Read the model definition and answer for the solid it produces. Units are mm, in the model's axes. Face numbers are marked on the shaded views. Coordinates: 2 decimals unless noted, no trailing zeros. Write each loop counter-clockwise with the first axis right and the second up, starting at its lowest first coordinate (ties: lowest second). Pieces come first, ordered by that corner, then holes.
1) The part is cut by section C-C (y = 56). Determine the outline of the cut face in (x, z).
2) Find the intervals of material crossed by line 1 (Y direction, x = 1.4, z = 8.2); line 2 (X direction, y = 48, z = 8.25); line 3 (Z direction, x = 15.25, y = 73), in increasing order.
3) Determine the mould class of the marked faces 1, 2, 3 and 4 for opening direction X: +X half, -X half, draft (parallel to the pull), parting line (faces both ways), or undercut.
4) Each of these flat-tipped pins is pushed along its axis until it touches: pin 1 Ø3.5 at (y, z) = (80, 8.2) entering from +X; pin 2 Ø1 at (x, z) = (26, 5.5) entering from +Y; pin 3 Ø1 at (x, y) = (22.5, 53) entering from +Z; pin 4 Ø1.6 at (x, z) = (25.5, 9.5) entering from -Y. Where does it stop, or does it pass through?
5) The part is cut by section A-A (z = 8.2). Determine the outline of the cut face in (x, y).
6) The part is cut by section D-D (x = 19). Determine the outline of the cut face in (y, z), then the cut area to 3 significant figures.
7) The part is cut by section B-B (y = 80). Determine the outline of the cut face in (x, z).
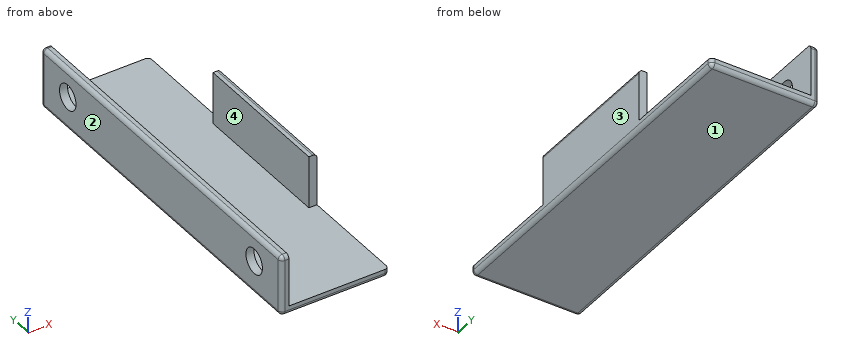
from build123d import *

# Parameters (mm, degrees)
SKETCH1_W           = 26.7
SKETCH1_H           = 90
BOSS_EXTRUDE1_DEPTH = 2
SKETCH2_W           = 2
SKETCH2_H           = 90
BOSS_EXTRUDE2_DEPTH = 12.9
SKETCH3_R           = 3.1
CUT_EXTRUDE1_DEPTH  = 96.052090982
FILLET1_R           = 1
FILLET2_R           = 1
FILLET3_R           = 1
FILLET6_R           = 1
FILLET7_R           = 1
FILLET8_R           = 1
CUT_EXTRUDE2_REACH  = 96.51
SKETCH5_W           = 12.9
SKETCH5_H           = 27


with BuildPart() as part:
    # Sketch1 → Boss-Extrude1 (new body)
    with BuildSketch(Plane.XY):
        with Locations((13.35, 45)):
            Rectangle(SKETCH1_W, SKETCH1_H)
    extrude(amount=BOSS_EXTRUDE1_DEPTH)

    # Sketch2 → Boss-Extrude2 (add)
    with BuildSketch(Plane.XY.offset(2)):
        with Locations((1, 45)):
            Rectangle(SKETCH2_W, SKETCH2_H)
        with Locations((25.7, 45)):
            Rectangle(SKETCH2_W, SKETCH2_H)
    extrude(amount=BOSS_EXTRUDE2_DEPTH)

    # Sketch3 → Cut-Extrude1 (cut, through all)
    with BuildSketch(Plane.ZY):
        with Locations((8.2, 10)):
            Circle(SKETCH3_R)
    cut_extrude1 = extrude(amount=-CUT_EXTRUDE1_DEPTH, mode=Mode.SUBTRACT)

    # Mirror1: Cut-Extrude1 across plane
    add(cut_extrude1.mirror(Plane.ZX.offset(45)), mode=Mode.SUBTRACT)

    # Fillet1
    fillet1_edges = [part.edges().sort_by_distance(p)[0] for p in [
        (13.35, 90, 0),
    ]]
    fillet(fillet1_edges, radius=FILLET1_R)

    # Fillet2
    fillet2_edges = [part.edges().sort_by_distance(p)[0] for p in [
        (0, 44.5, 0),
        (0, 89.707106781, 0.292893219),
        (0, 90, 7.95),
    ]]
    fillet(fillet2_edges, radius=FILLET2_R)

    # Fillet3
    fillet3_edges = [part.edges().sort_by_distance(p)[0] for p in [
        (26.7, 44.5, 0),
        (26.7, 89.707106781, 0.292893219),
        (26.7, 90, 7.95),
    ]]
    fillet(fillet3_edges, radius=FILLET3_R)

    # Fillet6
    fillet6_edges = [part.edges().sort_by_distance(p)[0] for p in [
        (13.35, 0, 0),
        (0.292893219, 0, 0.292893219),
        (26.7, 0, 7.95),
        (0, 0, 7.95),
        (26.407106781, 0, 0.292893219),
    ]]
    fillet(fillet6_edges, radius=FILLET6_R)

    # Fillet7
    fillet7_edges = [part.edges().sort_by_distance(p)[0] for p in [
        (1.5, 90, 14.9),
        (0, 45, 14.9),
        (0.292893219, 89.707106781, 14.9),
        (1.5, 0, 14.9),
        (0.292893219, 0.292893219, 14.9),
    ]]
    fillet(fillet7_edges, radius=FILLET7_R)

    # Fillet8
    fillet8_edges = [part.edges().sort_by_distance(p)[0] for p in [
        (25.2, 0, 14.9),
        (25.2, 90, 14.9),
        (26.407106781, 89.707106781, 14.9),
        (26.7, 45, 14.9),
        (26.407106781, 0.292893219, 14.9),
    ]]
    fillet(fillet8_edges, radius=FILLET8_R)

    # Cut-Extrude2: up to this face of the body (flat: up to its plane)
    cut_extrude2_end = Plane(part.part.faces().sort_by_distance((26.7, 45, 7.407866324))[0])
    # Sketch5 → Cut-Extrude2 (cut, up to the picked face)
    with BuildSketch(Plane.ZY.offset(-24.7), mode=Mode.PRIVATE) as cut_extrude2_sk1:
        with Locations((8.45, 76.5)):
            Rectangle(SKETCH5_W, SKETCH5_H)
    cut_extrude2_tool1 = split(extrude(cut_extrude2_sk1.sketch, amount=-CUT_EXTRUDE2_REACH, mode=Mode.PRIVATE), bisect_by=cut_extrude2_end, keep=Keep.BOTH, mode=Mode.PRIVATE)
    # Sketch5 → Cut-Extrude2 (cut, up to the picked face)
    with BuildSketch(Plane.ZY.offset(-24.7), mode=Mode.PRIVATE) as cut_extrude2_sk2:
        with Locations((8.45, 13.5)):
            Rectangle(SKETCH5_W, SKETCH5_H)
    cut_extrude2_tool2 = split(extrude(cut_extrude2_sk2.sketch, amount=-CUT_EXTRUDE2_REACH, mode=Mode.PRIVATE), bisect_by=cut_extrude2_end, keep=Keep.BOTH, mode=Mode.PRIVATE)
    add(cut_extrude2_tool1.solids().sort_by(Axis((24.7, 76.5, 8.45), (1, 0, 0)))[0], mode=Mode.SUBTRACT)
    add(cut_extrude2_tool2.solids().sort_by(Axis((24.7, 13.5, 8.45), (1, 0, 0)))[0], mode=Mode.SUBTRACT)


solid = part.part
Reported:
1. outline: (0, 1) arc R1 ccw to (1, 0) - (25.7, 0) arc R1 ccw to (26.7, 1) - (26.7, 13.9) arc R1 ccw to (25.7, 14.9) - (24.7, 14.9) - (24.7, 2) - (2, 2) - (2, 14.9) - (1, 14.9) arc R1 ccw to (0, 13.9) - close
2. line 1: y = 0 to 6.9, 13.1 to 76.9, 83.1 to 90
2. line 2: x = 0 to 2, 24.7 to 26.7
2. line 3: z = 0 to 2
3. face 1: draft
3. face 2: -X half
3. face 3: +X half
3. face 4: undercut
4. pin 1: passes through
4. pin 2: stops at y = 63
4. pin 3: stops at z = 2
4. pin 4: stops at y = 27
5. outline: (0, 1) arc R1 ccw to (1, 0) - (2, 0) - (2, 6.9) - (0, 6.9) - close; (0, 13.1) - (2, 13.1) - (2, 76.9) - (0, 76.9) - close; (0, 83.1) - (2, 83.1) - (2, 90) - (1, 90) arc R1 ccw to (0, 89) - close; (24.7, 27) - (26.7, 27) - (26.7, 63) - (24.7, 63) - close
6. outline: (0, 1) arc R1 ccw to (1, 0) - (89, 0) arc R1 ccw to (90, 1) - (90, 2) - (0, 2) - close
6. area: 180 mm2
7. outline: (0, 1) arc R1 ccw to (1, 0) - (25.7, 0) arc R1 ccw to (26.7, 1) - (26.7, 2) - (2, 2) - (2, 5.1) - (0, 5.1) - close; (0, 11.3) - (2, 11.3) - (2, 14.9) - (1, 14.9) arc R1 ccw to (0, 13.9) - close
